For this review, take the finished solid that the model builds, in its own axes (mm). Face numbers are marked on the shaded views. A direction names the side the tool comes from. Round coordinates to 2 decimals unless told otherwise and drop trailing zeros. Loops run counter-clockwise (first coordinate to the right, second up) from the corner with the lowest first, then second, coordinate; pieces in that order, holes last. Notation, with made-up numbers: M 74,20 L 129,20 A17 ccw 129,45 Z; hole C 65,31 d10. An arc over 180 degrees is marked long. One line per question, with ' | ' between items. Start each with the question number.
1) We need section B-B (z = -1.25). Give the boundary of the cut face in (x, y).
2) We need section C-C (x = -17). Give the boundary of the cut face in (y, z).
3) For probe 1 along Y at (x, z) = (-4.5, -6.5); probe 2 along X at (y, z) = (51.5, 0); probe 3 along Y at (x, z) = (-9, -13.75), list the stretches that pass through material, from the lowest coordinate up. Write a range as from..to.
4) For pin 1 Ø0.8 at (y, z) = (24.5, 9) entering from -X; pin 2 Ø8 at (x, y) = (-1, 16.5) entering from -Z; pin 3 Ø2 at (y, z) = (72.5, -10.5) entering from -X, all flat-tipped, find the tip position at first contact; note any pin that passes through.
5) We need section A-A (x = -24). Give the boundary of the cut face in (y, z), and give its area (3 significant figures).
6) Mouldability with a two-part tool opening along Z and no side actions: class the marked faces 4, 5 and 6 as pulls with the +Z half, pulls with the -Z half, needs draft (parallel to the pull), parting line crosses it, or undercut.
7) For the marked faces 1, 2 and 3, list the 3-axis set-ups (+Z, -Z, +X, -X, +Y, -Y) from which the entire face can be reached by the end or side of a thin tool; tool diameter is ignored.
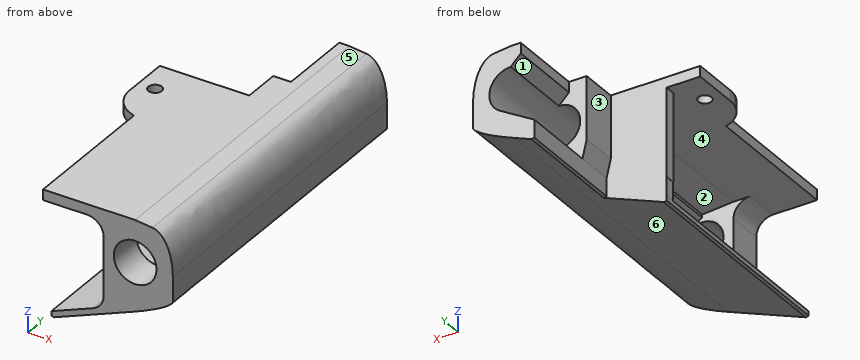
```python
from build123d import *
from OCP.BRepFilletAPI import BRepFilletAPI_MakeChamfer

# Parameters (mm, degrees)
SKETCH1_R           = 5.1
BOSS_EXTRUDE1_DEPTH = 80
CUT_EXTRUDE2_START  = -18
CUT_EXTRUDE2_DEPTH  = 18
CUT_EXTRUDE3_DEPTH  = 9
SKETCH8_R           = 1.6
CUT_EXTRUDE5_DEPTH  = 10
SKETCH10_W          = 12.5
SKETCH10_H          = 2.5
BOSS_EXTRUDE3_DEPTH = 21
CHAMFER1_SIZE       = 11.3
CHAMFER1_SIZE2      = 12.156054871
CHAMFER2_SIZE       = 0.4
CHAMFER2_SIZE2      = 0.751123796
SKETCH11_W          = 6
SKETCH11_H          = 34
CUT_EXTRUDE6_DEPTH  = 10
FILLET3_R           = 8
CUT_EXTRUDE7_START  = -50.5
CUT_EXTRUDE7_DEPTH  = 42
CHAMFER4_START      = 8.5
CHAMFER4_DEPTH      = 42
CHAMFER4_2_DEPTH    = 42
FILLET4_R           = 4


with BuildPart() as part:
    # Sketch1 → Boss-Extrude1 (new body)
    with BuildSketch(Plane(origin=(0, 0, 0), x_dir=(1, 0, 0), z_dir=(0, 1, 0))):
        Polygon((0, -10), (9, -9), (9, 8), (-20, 19.5), (-20, 18), (-7.5, 13.043103448), (-7.5, -7.5), (-28, -7.5), (-28, -10), align=None)
        with Locations(Location((0, 0, 0), (0, 0, 270))):
            Circle(SKETCH1_R, mode=Mode.SUBTRACT)
    extrude(amount=BOSS_EXTRUDE1_DEPTH)

    # Fillet1
    # a fillet whose section is not a circle: 10, 6 mm, written as the material it takes off along each edge
    with BuildSketch(Plane(origin=(9, -23.487180939, 9), x_dir=(-0.993883734673619, 0, 0.11043152607484658), z_dir=(0, 1, 0))) as fillet1_piece_1:
        with BuildLine():
            Bezier((4.925812314, 0), (0, 0), (-1.037490094, -9.337410844), weights=[1, 0.745128018, 1])
            Line((-1.037490094, -9.337410844), (0, 0))
            Line((0, 0), (4.925812314, 0))
        make_face()
    extrude(amount=126.974361879, mode=Mode.SUBTRACT)

    # Fillet2
    # a fillet whose section is not a circle: 12, 6 mm, written as the material it takes off along each edge
    with BuildSketch(Plane(origin=(9, -26.324436186, -8), x_dir=(-0.9295779033226579, 0, -0.368625720283123), z_dir=(0, 1, 0))) as fillet2_piece_1:
        with BuildLine():
            Bezier((10.529774474, 0), (0, 0), (-0.625160366, 1.576491357), weights=[1, 0.827232047, 1])
            Line((-0.625160366, 1.576491357), (0, 0))
            Line((0, 0), (10.529774474, 0))
        make_face()
    extrude(amount=132.648872372, mode=Mode.SUBTRACT)

    # Sketch5 → Cut-Extrude2 (cut)
    with BuildSketch(Plane(origin=(0, 80, 0), x_dir=(1, 0, 0), z_dir=(0, 1, 0)).offset(CUT_EXTRUDE2_START)):
        with BuildLine():
            Line((-40.382705662, 23.287650548), (-40.382705662, -15.07166092))
            Line((-40.382705662, -15.07166092), (-2.412422064, -15.07166092))
            Line((-2.412422064, -15.07166092), (-2.412422064, -7.512422064))
            Line((-2.412422064, -7.512422064), (0, -5.1))
            ThreePointArc((0, -5.1), (4.863777761, -1.534166188), (2.926213093, 4.176993768))
            Line((2.926213093, 4.176993768), (-5.637939913, 9.164476421))
            Line((-5.637939913, 9.164476421), (-5.637939913, 23.287650548))
            Line((-5.637939913, 23.287650548), (-40.382705662, 23.287650548))
        make_face()
    extrude(amount=CUT_EXTRUDE2_DEPTH, mode=Mode.SUBTRACT)

    # Sketch6 → Cut-Extrude3 (cut)
    with BuildSketch(Plane(origin=(0, 62, 0), x_dir=(1, 0, 0), z_dir=(0, 1, 0))):
        Polygon((-6.637939913, -10), (-28, -10), (-28, 21.40414119), (-6.637939913, 21.40414119), (-5.637939913, 21.40414119), (-5.637939913, 9.164476421), (-6.637939913, 4.905415269), align=None)
    extrude(amount=-CUT_EXTRUDE3_DEPTH, mode=Mode.SUBTRACT)

    # Sketch8 → Cut-Extrude5 (cut)
    with BuildSketch(Plane.XY.offset(10)):
        with Locations((-24, 45)):
            Circle(SKETCH8_R)
    extrude(amount=-CUT_EXTRUDE5_DEPTH, mode=Mode.SUBTRACT)

    # Sketch10 → Boss-Extrude3 (add)
    with BuildSketch(Plane(origin=(0, 0, 7.5), x_dir=(-1, 0, 0), z_dir=(0, 0, -1))):
        with Locations((13.75, 51.75)):
            Rectangle(SKETCH10_W, SKETCH10_H)
    extrude(amount=BOSS_EXTRUDE3_DEPTH)

    # Chamfer1
    chamfer1_edges = [part.edges().sort_by_distance(p)[0] for p in [
        (-8.652173913, 51.75, -13.5),
    ]]
    chamfer1_side = [part.faces().sort_by_distance(p)[0] for p in [
        (-14.326086957, 51.75, -13.5),
    ]]
    chamfer(chamfer1_edges, length=CHAMFER1_SIZE, length2=CHAMFER1_SIZE2, reference=chamfer1_side[0])

    # Chamfer2: one chamfer whose edges measure the first distance from different faces: ONE call of the kernel's chamfer builder (chamfer() names one face for all edges)
    chamfer2_edges_1 = [part.edges().sort_by_distance(p)[0] for p in [
        (-5.637939913, 66.5, -13.80470031),
    ]]
    chamfer2_side_1 = [part.faces().sort_by_distance(p)[0] for p in [
        (-5.637939913, 66.5, -11.484588366),
    ]]
    chamfer2_edges_2 = [part.edges().sort_by_distance(p)[0] for p in [
        (-20, 26.5, -19.5),
    ]]
    chamfer2_side_2 = [part.faces().sort_by_distance(p)[0] for p in [
        (-20, 26.5, -18.75),
    ]]
    chamfer2 = BRepFilletAPI_MakeChamfer(part.part.solid().wrapped)
    for e in chamfer2_edges_1:
        chamfer2.Add(CHAMFER2_SIZE, CHAMFER2_SIZE2, e.wrapped, chamfer2_side_1[0].wrapped)  # the first distance lies on this face
    for e in chamfer2_edges_2:
        chamfer2.Add(CHAMFER2_SIZE, CHAMFER2_SIZE2, e.wrapped, chamfer2_side_2[0].wrapped)  # the first distance lies on this face
    add(Compound.cast(chamfer2.Shape()), mode=Mode.REPLACE)

    # Sketch11 → Cut-Extrude6 (cut)
    with BuildSketch(Plane(origin=(0, 0, 7.5), x_dir=(-1, 0, 0), z_dir=(0, 0, -1))):
        with Locations((25, 17)):
            Rectangle(SKETCH11_W, SKETCH11_H)
    extrude(amount=-CUT_EXTRUDE6_DEPTH, mode=Mode.SUBTRACT)

    # Fillet3
    # the kernel refuses this fillet: 8 mm, written as the material it takes off along each edge
    with BuildSketch(Plane(origin=(-28, 34, -11.864916731), x_dir=(0, 1, 0), z_dir=(0, 0, 1))) as fillet3_piece_1:
        with BuildLine():
            CenterArc((7.745966692, -8), FILLET3_R, 90, 75.522487814)
            Line((0, -6), (-0.154919334, -5.96))
            ThreePointArc((-0.154919334, -5.96), (-0.16, -3), (-0.16, 0))
            Line((-0.16, 0), (0, 0.16))
            Line((0, 0.16), (7.745966692, 0.16))
            Line((7.745966692, 0.16), (7.745966692, 0))
        make_face()
    extrude(amount=41.229833462, mode=Mode.SUBTRACT)

    # Sketch12 → Cut-Extrude7 (cut)
    with BuildSketch(Plane.XZ.offset(CUT_EXTRUDE7_START)):
        Polygon((-7.5, -13.043103448), (0, -9.648284322), (0, 6.91148674), (-7.5, 7.5), align=None)
    extrude(amount=CUT_EXTRUDE7_DEPTH, mode=Mode.SUBTRACT)

    # Chamfer3
    # the kernel refuses this chamfer: 10 mm, written as the material it takes off along each edge
    with BuildSketch(Plane(origin=(0, 50.5, -5.1), x_dir=(0.9352222959192602, 0, 0.3540610924904171), z_dir=(0, -1, 0))) as chamfer3_piece_1_section:
        with BuildLine():
            Line((3.894265856, 0.282842712), (-2.483031603, -6.094454747))
            Line((-2.483031603, -6.094454747), (-2.670076063, -6.023642528))
            ThreePointArc((-2.670076063, -6.023642528), (-1.351695644, -3.005514942), (-0.187044459, 0.070812218))
            Line((-0.187044459, 0.070812218), (0.070812218, 0.187044459))
            ThreePointArc((0.070812218, 0.187044459), (1.955367921, -0.128080347), (3.823453637, 0.469887172))
            Line((3.823453637, 0.469887172), (3.894265856, 0.282842712))
        make_face()
    chamfer3_piece_1 = extrude(amount=42, mode=Mode.PRIVATE)
    chamfer3_piece_1 = split(chamfer3_piece_1, bisect_by=Plane(origin=(1.70866642, 50.5, -8.874869196), z_dir=(-0.4123656941532171, 0, 0.9110184050201925)), keep=Keep.TOP, mode=Mode.PRIVATE)
    add(chamfer3_piece_1, mode=Mode.SUBTRACT)

    # Chamfer4: read off the stored shape, not the designer's step
    # Chamfer4 outline → Chamfer4 (cut)
    with BuildSketch(Plane(origin=(0, 0, 0), x_dir=(1, 0, 0), z_dir=(0, 1, 0)).offset(CHAMFER4_START)):
        with BuildLine():
            Line((0, -5.1), (0, -6.228017105))
            Line((0, -6.228017105), (2.673318305, -4.343198043))
            ThreePointArc((2.673318305, -4.343198043), (1.389188609, -4.907153453), (0, -5.1))
        make_face()
    extrude(amount=CHAMFER4_DEPTH, mode=Mode.SUBTRACT)

    # Chamfer4 2 outline → Chamfer4 2 (add)
    with BuildSketch(Plane(origin=(0, 0, 0), x_dir=(1, 0, 0), z_dir=(0, 1, 0)).offset(CHAMFER4_START)):
        with BuildLine():
            Line((3.192787517, -3.976947054), (2.673318305, -4.343198043))
            ThreePointArc((2.673318305, -4.343198043), (2.938764081, -4.168172942), (3.192787517, -3.976947054))
        make_face()
    extrude(amount=CHAMFER4_2_DEPTH)

    # Fillet4
    # the kernel refuses this fillet: 4 mm, written as the material it adds along each edge
    with BuildSketch(Plane(origin=(-7.5, 0, 7.5), x_dir=(-1, 0, 0), z_dir=(0, 1, 0))) as fillet4_piece_1:
        with BuildLine():
            CenterArc((FILLET4_R, -FILLET4_R), FILLET4_R, 90, 90)
            Line((0, -FILLET4_R), (0, 0))
            Line((0, 0), (FILLET4_R, 0))
        make_face()
    extrude(amount=8.5)
    with BuildSketch(Plane(origin=(-7.5, 0, -13.043103448), x_dir=(-0.9295779033226581, 0, -0.3686257202831227), z_dir=(0, 1, 0))) as fillet4_piece_2:
        with BuildLine():
            CenterArc((FILLET4_R * 0.679205344125, FILLET4_R), FILLET4_R, 201.630886837, 68.369113163)
            Line((-FILLET4_R * 0.250372559198, FILLET4_R * 0.631374279717), (0, 0))
            Line((0, 0), (FILLET4_R * 0.679205344125, 0))
        make_face()
    extrude(amount=8.5)


solid = part.part
```
Answers below:
1) outline: M -20,50.5 L -4.94,50.5 L -4.94,62 L -6.64,62 L -6.64,53 L -20,53 Z; M -7.5,0 L -4.94,0 L -4.94,8.5 L -7.5,8.5 Z; M 4.94,0 L 9,0 L 9,80 L 4.94,80 Z
2) outline: M 0,-18.31 L 53,-18.31 L 53,10 L 0,10 L 0,7.5 L 50.5,7.5 L 50.5,-16.81 L 0,-16.81 Z
3) probe 1: 0..8.5, 50.5..62 | probe 2: -20..-5.1, 5.1..9 | probe 3: 0..53
4) pin 1: x = -22 | pin 2: z = -13.55 | pin 3: x = -5.64
5) outline: M 34.82,7.5 L 43.4,7.5 L 43.4,10 L 34.82,10 Z; M 46.6,7.5 L 53,7.5 L 53,10 L 46.6,10 Z | area: 37.5 mm^2
6) face 4: undercut | face 5: pulls with the +Z half | face 6: pulls with the -Z half
7) face 1: -X, +Y | face 2: -X | face 3: +Z, -Z, -X, +Y
